Build history of the part. All positions in model axes, mm. Give positions to 0.01 mm unless a question says otherwise; leave off trailing zeros. Loops run counter-clockwise (first coordinate to the right, second up) from the corner with the lowest first, then second, coordinate; pieces in that order, holes last. Notation, with made-up numbers: (-34.5, -18) -> (10.5, -18) arc R18 cw to (10.5, -2) -> close; hole circle Ø9 at (-33.5, 80). An arc over 180 degrees is marked (long way). Answer as a JSON object with one key per item and string values. Group by question number.
Q1. Drop flat-ended pins along their axis: pin 1 (8 mm diameter, centred on x = 35.5, y = 20.5, fed in from +Z); pin 2 (1.5 mm diameter, centred on y = 21, z = -3.5, fed in from -X); pin 3 (1.5 mm diameter, centred on y = 24.5, z = -4, fed in from -X). Give the stop position or say it passes through.
Q2. Two-plate mould, pull along Y, no slides. Class faces 1 (the cylindrical face through (1.81, 22.54, -1.91)), 2 (the cylindrical face through (14.38, 18.35, -3.13)), 3 (the flat face through (69, 44.45, -3)): pulls with the +Y half, pulls with the -Y half, needs draft (parallel to the pull), parting line crosses it, or undercut.
Q3. Wall check: probe 1 along Y at (x, z) = (15.24, -2.5); probe 2 along Y at (x, z) = (16.5, -3.5); probe 3 along X at (y, z) = (30, -6). Give the ranges that are in metal, low to high. Write a range as from..to.
Q4. Band-saw the part on A-A, the plane x = 15.24. Write the cut outline in (y, z).
from build123d import *

# Parameters (mm, degrees)
SKETCH1_W           = 139.7
SKETCH1_H           = 6.35
BOSS_EXTRUDE1_DEPTH = 44.45
FILLET1_R           = 6.35
SKETCH4_R           = 3.96875
CUT_EXTRUDE2_DEPTH  = 254


with BuildPart() as part:
    # Sketch1 → Boss-Extrude1 (new body)
    with BuildSketch(Plane(origin=(0, 0, 0), x_dir=(1, 0, 0), z_dir=(0, 1, 0))):
        with Locations((69.85, 3.175)):
            Rectangle(SKETCH1_W, SKETCH1_H)
    extrude(amount=BOSS_EXTRUDE1_DEPTH)

    # Fillet1
    fillet1_edges = [part.edges().sort_by_distance(p)[0] for p in [
        (0, 22.225, 0),
    ]]
    fillet(fillet1_edges, radius=FILLET1_R - 0.0001)  # a hair under: the kernel refuses the full size

    # Sketch4 → Cut-Extrude2 (cut)
    with BuildSketch(Plane(origin=(69.948790088, 1.415162488, 0), x_dir=(1, 0, 0), z_dir=(0, 0, 1))):
        with Locations((-54.708790088, 20.809837512)):
            Circle(SKETCH4_R)
    extrude(amount=-CUT_EXTRUDE2_DEPTH, mode=Mode.SUBTRACT)


solid = part.part
Worked answers:
{
 "1": {"pin 1": "z = 0", "pin 2": "x = 0.36", "pin 3": "x = 0.2"},
 "2": {"face 1": "needs draft", "face 2": "undercut", "face 3": "pulls with the +Y half"},
 "3": {"probe 1": "0..18.26, 26.19..44.45", "probe 2": "0..18.46, 25.99..44.45", "probe 3": "0.01..139.7"},
 "4": {"outline": "(0, -6.35) -> (18.26, -6.35) -> (18.26, 0) -> (0, 0) -> close; (26.19, -6.35) -> (44.45, -6.35) -> (44.45, 0) -> (26.19, 0) -> close"}
}
